Here's the drawing with two shaded views (mm, measured from the low corner). I have some questions. A direction names the side the tool comes from. Give positions to 0.01 mm unless a question says otherwise; leave off trailing zeros. Loops run counter-clockwise (first coordinate to the right, second up) from the corner with the lowest first, then second, coordinate; pieces in that order, holes last. Notation, with made-up numbers: (88, 34) - (142, 34) arc R22 cw to (142, 58) - close; hole circle Ø1 at (-2, 6.25). An arc over 180 degrees is marked (long way). Write each question's results on one line, items separated by ' | '. Start each with the question number.
1) If we mould it in two halves opening along Y, with no side actions, what happens to the marked faces 1, 2 and 3? For each: +Y half, -Y half, draft (parallel to the pull), parting line (faces both ways), or undercut.
2) I'm going to push flat-ended pins straight in: pin 1 (3 mm diameter, centred on x = 10, y = 6.5, fed in from +Z); pin 2 (4 mm diameter, centred on x = 6.5, y = 13.5, fed in from -Z); pin 3 (8 mm diameter, centred on y = 2, z = 9, fed in from -X). Where does each tip first touch, or does it pass through?
3) If I drill on probe 1 along Z at (x, y) = (3.5, 9); probe 2 along Z at (x, y) = (5, 2.75); probe 3 along X at (y, z) = (11, 14), over which ranges is the centre line in solid material (lowest first)? Write a range as [from, to].
4) I want a section at B-B, the plane z = 22. Write out the boundary of the cut face in (x, y).
5) I want a section at D-D, the plane z = 5. Write out the boundary of the cut face in (x, y), and give its area (3 significant figures).
6) I want a section at C-C, the plane x = 14.5. Write out the boundary of the cut face in (y, z).
7) On a 3-axis mill with a long thin cutter (end or side, diameter ignored), from which of +Z, -Z, +X, -X, +Y, -Y can I reach the whole of each face in a straight line? I mean the marked faces 4, 5 and 6. Say none if no direction works.
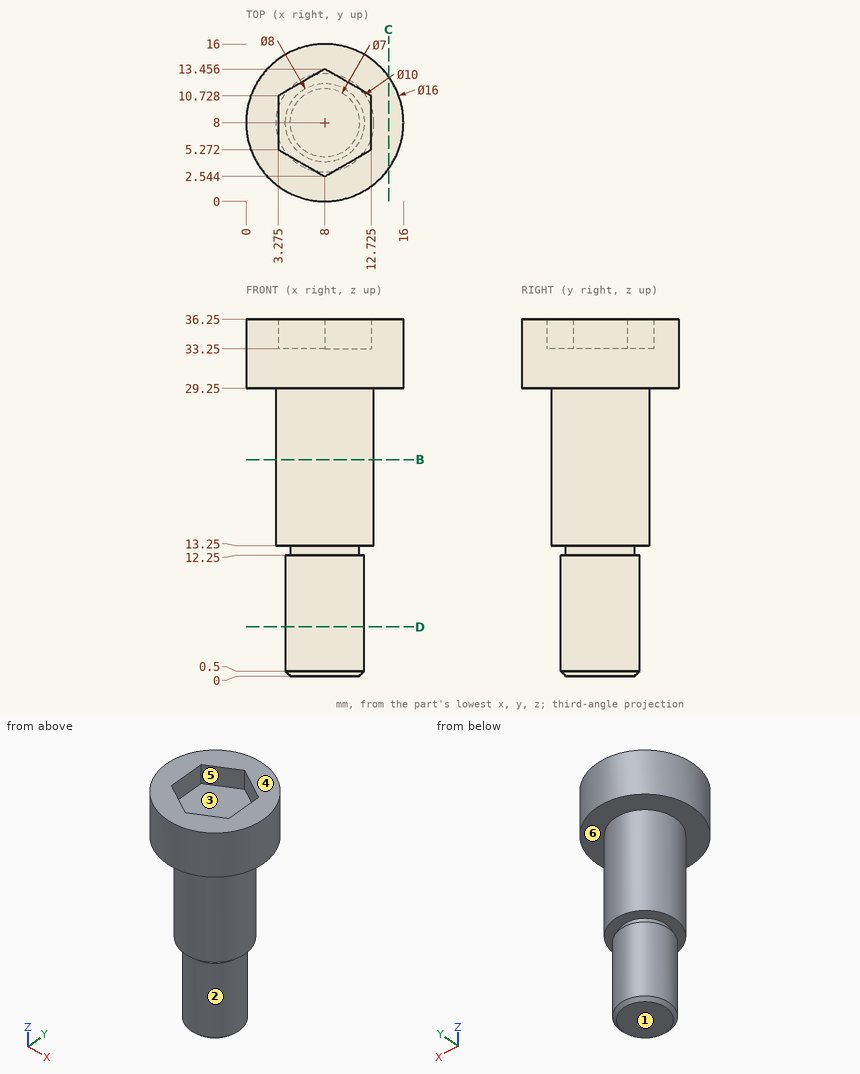
Answers:
1) face 1: draft | face 2: parting line | face 3: undercut
2) pin 1: stops at z = 33.25 | pin 2: stops at z = 0.2 | pin 3: stops at x = 4.54
3) probe 1: z = [13.25, 33.25] | probe 2: z = [29.25, 36.25] | probe 3: x = [4, 12]
4) outline: circle Ø10 at (8, 8)
5) outline: circle Ø8 at (8, 8) | area: 50.3 mm2
6) outline: (3.34, 29.25) - (12.66, 29.25) - (12.66, 36.25) - (3.34, 36.25) - close
7) face 4: +Z, +X, -X, +Y, -Y | face 5: +Z | face 6: -Z
